from build123d import *

# Parameters (mm, degrees)
SKETCH_2_R      = 1.05
EXTRUDE_1_DEPTH = 2
FILLET_1_R      = 1


with BuildPart() as part:
    # 草图2 → 凸台-拉伸1 (new body)
    with BuildSketch(Plane(origin=(0, 0, 0), x_dir=(1, 0, 0), z_dir=(0, 1, 0))):
        Polygon((-36, 17.5), (-32, 13.5), (32, 13.5), (36, 17.5), (40, 17.5), (40, -17.5), (36, -17.5), (32, -13.5), (-32, -13.5), (-36, -17.5), (-40, -17.5), (-40, 17.5), align=None)
        with Locations(Location((-37.5, 15, 0), (0, 0, 270))):
            Circle(SKETCH_2_R, mode=Mode.SUBTRACT)
        with Locations(Location((37.5, 15, 0), (0, 0, 270))):
            Circle(SKETCH_2_R, mode=Mode.SUBTRACT)
        with Locations(Location((37.5, -15, 0), (0, 0, 270))):
            Circle(SKETCH_2_R, mode=Mode.SUBTRACT)
        with Locations(Location((-37.5, -15, 0), (0, 0, 270))):
            Circle(SKETCH_2_R, mode=Mode.SUBTRACT)
        Polygon((30.642857143, 10.5), (0, 1.5625), (-30.642857143, 10.5), align=None, mode=Mode.SUBTRACT)
        Polygon((-30.642857143, -10.5), (0, -1.5625), (30.642857143, -10.5), align=None, mode=Mode.SUBTRACT)
        Polygon((-36, 8.9375), (-5.357142857, 0), (-36, -8.9375), align=None, mode=Mode.SUBTRACT)
        Polygon((36, -8.9375), (36, 8.9375), (5.357142857, 0), align=None, mode=Mode.SUBTRACT)
    extrude(amount=EXTRUDE_1_DEPTH)

    # 圆角1
    fillet_1_edges = [part.edges().sort_by_distance(p)[0] for p in [
        (-30.642857143, 1, 10.5),
        (30.642857143, 1, 10.5),
        (0, 1, 1.5625),
        (36, 1, 8.9375),
        (36, 1, -8.9375),
        (5.357142857, 1, 0),
        (-36, 1, -8.9375),
        (-36, 1, 8.9375),
        (-5.357142857, 1, 0),
        (-40, 1, 17.5),
        (-40, 1, -17.5),
        (-36, 1, -17.5),
        (-32, 1, -13.5),
        (32, 1, -13.5),
        (36, 1, -17.5),
        (40, 1, -17.5),
        (40, 1, 17.5),
        (36, 1, 17.5),
        (32, 1, 13.5),
        (-32, 1, 13.5),
        (-36, 1, 17.5),
        (-30.642857143, 1, -10.5),
        (0, 1, -1.5625),
        (30.642857143, 1, -10.5),
    ]]
    fillet(fillet_1_edges, radius=FILLET_1_R)


solid = part.part
For this review, take the finished solid that the model builds, in its own axes (mm). A direction names the side the tool comes from. Coordinates: 2 decimals unless noted, no trailing zeros. Write each loop counter-clockwise with the first axis right and the second up, starting at its lowest first coordinate (ties: lowest second). Pieces come first, ordered by that corner, then holes. Notation, with made-up numbers: (40.25, -30.75) -> (63.25, -30.75) arc R12 cw to (63.25, -19.75) -> close; hole circle Ø7 at (30.25, 80.5). An arc over 180 degrees is marked (long way). Write each question's results on one line, items separated by ' | '. Start each with the question number.
1) Wall thickness on L1, parallel to Z at x = 0, y = 0.9; L2, parallel to X at y = 1.45, z = -15; L3, parallel to Z at x = 11, y = 0.6: over which ranges is each line inside the solid? List them lowest first. Write a range as [from, to].
2) For faces 1 (the face through (34, 1, 15.5)), 2 (the face through (-40, 1, 0)), 3 (the face through (-21.5, 0.99, 4.71)), list the 3-axis set-ups (+Z, -Z, +X, -X, +Y, -Y) from which the entire face can be reached by the end or side of a thin tool; tool diameter is ignored.
3) Insertion check: pin 1 (12 mm diameter, centred on x = -12, z = -6.5, fed in from -Y); pin 2 (1 mm diameter, centred on x = -9.5, y = 1, fed in from +Z); pin 3 (0.6 mm diameter, centred on x = -6.5, y = 1, fed in from -Z). Each pin has a flat end and moves straight along its axis. Give the tip position at first contact, or say it passes through.
4) The part is to be moulded in two halves that separate along Z. For faces 4 (the face through (38, 1, -17.5)), 5 (the face through (1, 2, 0)), 6 (the face through (0, 1, -10.5)), 7 (the face through (-12.27, 0.99, 5.14)), say which applies: +Z half, -Z half, draft (parallel to the pull), parting line (faces both ways), or undercut.
5) Consider section A-A (z = -15). Write out the cut boundary in (x, y), plus the area to 3 significant figures.
6) Consider section B-B (x = -37.5). Write out the cut boundary in (y, z), plus the area to 3 significant figures.
7) Consider section D-D (y = 0.45). Give the number of separate pieces and of enclosed holes in the cut face, plus the area to 3 significant figures.
8) Consider section C-C (x = 29). Write out the cut boundary in (y, z), plus the area to 3 significant figures.
Geometry says:
1) L1: [-13.5, -10.5], [-1.6, 1.6], [10.5, 13.5] | L2: [-40, -38.55], [-36.45, -33.5], [33.5, 36.45], [38.55, 40] | L3: [-13.5, -10.5], [-4.77, -1.65], [1.65, 4.77], [10.5, 13.5]
2) face 1: +Z, +Y, -Y | face 2: +Z, -Z, -X, +Y, -Y | face 3: +Y, -Y
3) pin 1: y = 0 | pin 2: z = 13.5 | pin 3: z = -13.5
4) face 4: -Z half | face 5: draft | face 6: undercut | face 7: undercut
5) outline: (-40, 0) -> (-38.55, 0) -> (-38.55, 2) -> (-40, 2) -> close; (-36.45, 0) -> (-33.5, 0) -> (-33.5, 2) -> (-36.45, 2) -> close; (33.5, 0) -> (36.45, 0) -> (36.45, 2) -> (33.5, 2) -> close; (38.55, 0) -> (40, 0) -> (40, 2) -> (38.55, 2) -> close | area: 17.6 mm^2
6) outline: (0, -17.5) -> (2, -17.5) -> (2, -16.05) -> (0, -16.05) -> close; (0, -13.95) -> (2, -13.95) -> (2, 13.95) -> (0, 13.95) -> close; (0, 16.05) -> (2, 16.05) -> (2, 17.5) -> (0, 17.5) -> close | area: 61.6 mm^2
7) separate pieces: 1 | enclosed holes: 8 | area: 1,170 mm^2
8) outline: (0, -13.5) -> (2, -13.5) -> (2, -6.9) -> (0, -6.9) -> close; (0, 6.9) -> (2, 6.9) -> (2, 13.5) -> (0, 13.5) -> close | area: 26.4 mm^2
